```python
from build123d import *

# Parameters (mm, degrees)
SKETCH1_R           = 31.75
SKETCH1_R_2         = 4.000000128
BOSS_EXTRUDE1_DEPTH = 1.27
BOSS_EXTRUDE3_DEPTH = 2.54
SKETCH3_R           = 2.5527
CUT_EXTRUDE1_DEPTH  = 3.54
CUT_EXTRUDE2_DEPTH  = 3.54
CIRPATTERN1_COUNT   = 4


with BuildPart() as part:
    # Sketch1 → Boss-Extrude1 (new body, symmetric)
    with BuildSketch(Plane(origin=(0, 0, 0), x_dir=(1, 0, 0), z_dir=(0, 1, 0))):
        Circle(SKETCH1_R)
        Circle(SKETCH1_R_2, mode=Mode.SUBTRACT)
    extrude(amount=BOSS_EXTRUDE1_DEPTH, both=True)

    # Sketch2 → Boss-Extrude3 (add, through all)
    with BuildSketch(Plane(origin=(0, 1.27, 0), x_dir=(1, 0, 0), z_dir=(0, 1, 0))):
        with BuildLine():
            Line((-2.667, -2.981125966), (-2.667, 2.981125966))
            ThreePointArc((-2.667, 2.981125966), (-4.000000128, 0), (-2.667, -2.981125966))
        make_face()
    extrude(amount=-BOSS_EXTRUDE3_DEPTH)

    # Sketch3 → Cut-Extrude1 (cut, through all)
    with BuildSketch(Plane(origin=(0, 1.27, 0), x_dir=(1, 0, 0), z_dir=(0, 1, 0))):
        with Locations((0, 25.4)):
            Circle(SKETCH3_R)
    cut_extrude1 = extrude(amount=-CUT_EXTRUDE1_DEPTH, mode=Mode.SUBTRACT)

    # Sketch4 → Cut-Extrude2 (cut, through all)
    with BuildSketch(Plane(origin=(0, 1.27, 0), x_dir=(1, 0, 0), z_dir=(0, 1, 0))):
        with BuildLine():
            Line((3.81, 8.729806699), (3.81, 20.32))
            ThreePointArc((3.81, 20.32), (5.788743237, 22.789836838), (6.329647384, 25.908))
            ThreePointArc((6.329647384, 25.908), (18.858537854, 18.858537854), (25.908, 6.329647384))
            ThreePointArc((25.908, 6.329647384), (22.789836838, 5.788743237), (20.32, 3.81))
            Line((20.32, 3.81), (8.729806699, 3.81))
            ThreePointArc((8.729806699, 3.81), (6.735192091, 6.735192091), (3.81, 8.729806699))
        make_face()
    cut_extrude2 = extrude(amount=-CUT_EXTRUDE2_DEPTH, mode=Mode.SUBTRACT)

    # CirPattern1: Cut-Extrude1, Cut-Extrude2 ×4 about axis
    cirpattern1_axis = Axis((0, 0, 0), (0, 1, 0))
    for i in range(1, CIRPATTERN1_COUNT):
        add(cut_extrude1.rotate(cirpattern1_axis, i * 360 / CIRPATTERN1_COUNT), mode=Mode.SUBTRACT)
        add(cut_extrude2.rotate(cirpattern1_axis, i * 360 / CIRPATTERN1_COUNT), mode=Mode.SUBTRACT)


solid = part.part
```
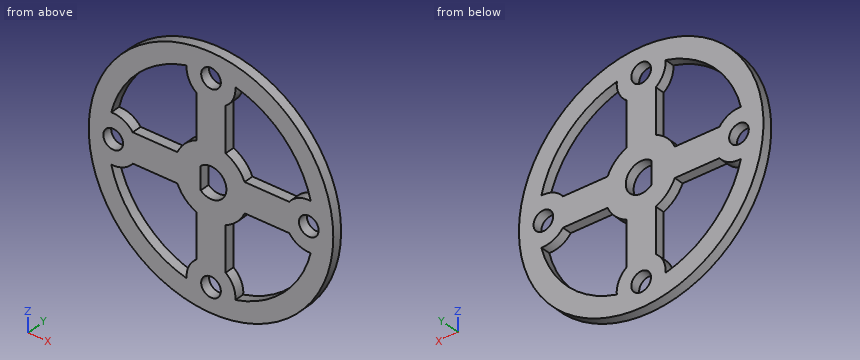
Check sheet for the modelled part. Datum: model origin and axes. Units: mm. Coordinates: 2 decimals unless noted, no trailing zeros. Write each loop counter-clockwise with the first axis right and the second up, starting at its lowest first coordinate (ties: lowest second). Pieces come first, ordered by that corner, then holes. Notation, with made-up numbers: (-6, 47) -> (30, 47) arc R29 cw to (30, 84) -> close; hole circle Ø3 at (21, 47.25). An arc over 180 degrees is marked (long way). Use a Markdown table: item, result.
1. Sectioned sample at D-D (x = 15). Enter the section's corners in (y, z).
Reported:
| item | result |
|---|---|
| outline | (-1.27, -27.98) -> (1.27, -27.98) -> (1.27, -22.05) -> (-1.27, -22.05) -> close; (-1.27, -3.81) -> (1.27, -3.81) -> (1.27, 3.81) -> (-1.27, 3.81) -> close; (-1.27, 22.05) -> (1.27, 22.05) -> (1.27, 27.98) -> (-1.27, 27.98) -> close |
2. Scan lines: line 1 along X through (y, z) = (-0.55, 0); line 2 along Z through (x, y) = (0, 0); line 3 along Z through (x, y) = (7, -0.8). Record each from-to range of solid material in increasing order.
Reported:
| item | result |
|---|---|
| line 1 | x = -31.75 to -27.95, -22.85 to -2.67, 4 to 22.85, 27.95 to 31.75 |
| line 2 | z = -31.75 to -27.95, -22.85 to -4, 4 to 22.85, 27.95 to 31.75 |
| line 3 | z = -30.97 to -25.73, -6.46 to 6.46, 25.73 to 30.97 |
3. Sectioned sample at C-C (y = -0.65). Give the number of separate pieces and of enclosed holes in the cut face, plus the area to 3 significant figures.
Reported:
| item | result |
|---|---|
| separate pieces | 1 |
| enclosed holes | 9 |
| area | 1,710 mm2 |
4. Sectioned sample at A-A (x = 0). Enter the section's corners in (y, z).
Reported:
| item | result |
|---|---|
| outline | (-1.27, -31.75) -> (1.27, -31.75) -> (1.27, -27.95) -> (-1.27, -27.95) -> close; (-1.27, -22.85) -> (1.27, -22.85) -> (1.27, -4) -> (-1.27, -4) -> close; (-1.27, 4) -> (1.27, 4) -> (1.27, 22.85) -> (-1.27, 22.85) -> close; (-1.27, 27.95) -> (1.27, 27.95) -> (1.27, 31.75) -> (-1.27, 31.75) -> close |
5. Sectioned sample at B-B (z = 0). Enter the section's corners in (x, y).
Reported:
| item | result |
|---|---|
| outline | (-31.75, -1.27) -> (-27.95, -1.27) -> (-27.95, 1.27) -> (-31.75, 1.27) -> close; (-22.85, -1.27) -> (-2.67, -1.27) -> (-2.67, 1.27) -> (-22.85, 1.27) -> close; (4, -1.27) -> (22.85, -1.27) -> (22.85, 1.27) -> (4, 1.27) -> close; (27.95, -1.27) -> (31.75, -1.27) -> (31.75, 1.27) -> (27.95, 1.27) -> close |
6. Go/stop test with flat-tipped pins: pin 1 Ø0.8 at (x, y) = (-15, -0.5) entering from -Z; pin 2 Ø1.3 at (y, z) = (0, 14) entering from +X; pin 3 Ø1.3 at (x, y) = (12, 0.5) entering from -Z; pin 4 Ø7 at (x, z) = (0, 0) entering from -Y. Record where each tip stops, or that it passes through.
Reported:
| item | result |
|---|---|
| pin 1 | stops at z = -28.19 |
| pin 2 | stops at x = 28.81 |
| pin 3 | stops at z = -29.65 |
| pin 4 | stops at y = -1.27 |
